```python
from build123d import *

# Parameters (mm, degrees)
CHAMFER1_SIZE = 0.2


with BuildPart() as part:
    # Sketch1 → Revolve1 (revolve)
    with BuildSketch(Plane.XY, mode=Mode.PRIVATE) as revolve1_sk:
        with BuildLine():
            Line((2.38125, 3.495554014), (2.38125, 2.495554014))
            Line((2.38125, 2.495554014), (4.7625, 2.495554014))
            Line((4.7625, 2.495554014), (4.7625, 0))
            Line((4.7625, 0), (2.38125, 0))
            Line((2.38125, 0), (2.38125, -11.43))
            Line((2.38125, -11.43), (0, -11.43))
            Line((0, -11.43), (0, 12.3825))
            ThreePointArc((0, 12.3825), (4.600221748, 8.852625702), (2.38125, 3.495554014))
        make_face()
    revolve(revolve1_sk.sketch.rotate(Axis((0, 48.717648678, 0), (0, -1, 0)), 180), axis=Axis((0, 48.717648678, 0), (0, -1, 0)))  # turned: the seam where the file's is

    # Chamfer1
    chamfer1_edges = [part.edges().sort_by_distance(p)[0] for p in [
        (2.38125, -11.43, 0),
        (4.7625, 0, 0),
        (4.7625, 2.495554014, 0),
    ]]
    chamfer(chamfer1_edges, length=CHAMFER1_SIZE)


solid = part.part
```
Design review of the part built by this model. Coordinates are the model's own, in mm. A direction names the side the tool comes from. Round coordinates to 2 decimals unless told otherwise and drop trailing zeros. Write each loop counter-clockwise with the first axis right and the second up, starting at its lowest first coordinate (ties: lowest second). Pieces come first, ordered by that corner, then holes. Notation, with made-up numbers: (28, 56.25) -> (55, 56.25) arc R16 ccw to (55, 76.25) -> close; hole circle Ø10 at (29, 10.25). An arc over 180 degrees is marked (long way). Write item = value, one per line. Start each with the question number.
1) Take a section at D-D, the plane y = 2. State the section outline as (x, z) points (1 decimal).
2) Clearance check with flat-ended pins moving along their axes: pin 1 (1 mm diameter, centred on x = -1.5, z = -3, fed in from -Y); pin 2 (3 mm diameter, centred on y = -7, z = -1, fed in from +X); pin 3 (2 mm diameter, centred on y = 5.5, z = 3, fed in from -X). State where each tip first meets the part, or that it passes through.
3) Wall thickness on probe 1 along Y at (x, z) = (-3, 2); probe 2 along Y at (x, z) = (2.75, -2.5); probe 3 along Z at (x, y) = (-2.5, 9.5): over which ranges is each line inside the solid? List them lowest first. Write a range as from..to.
4) Tool access review of faces 1 (the face through (2, 2.496, 2)), 2 (the face through (1.03, 1.23, 4.65)), 3 (the face through (-2, 0, 2)): name each direction out of +Z, -Z, +X, -X, +Y, -Y from which nothing blocks a thin tool from reaching the whole face with its end or side.
5) Take a section at C-C, the plane y = -2. State the section outline as (x, z) points, plus the area to 3 significant figures.
6) Mouldability with a two-part tool opening along Y and no side actions: class faces 4 (the face through (0, -11.43, 0)), 5 (the face through (0.516, 2.989, 2.325)), 6 (the face through (0.516, -5.694, 2.325)) as +Y half, -Y half, draft (parallel to the pull), parting line (faces both ways), or undercut.
Results list:
q1.outline = circle Ø9.5 at (0, 0)
q2.pin_1 = 0
q2.pin_2 = 2.38
q2.pin_3 = -3.94
q3.probe_1 = 0..2.5, 4.51..10.73
q3.probe_2 = 0..2.5, 4.64..10.6
q3.probe_3 = -3.59..3.59
q4.face_1 = none
q4.face_2 = +Y, -Y
q4.face_3 = -Y
q5.outline = circle Ø4.76 at (0, 0)
q5.area = 17.8 mm²
q6.face_4 = -Y half
q6.face_5 = undercut
q6.face_6 = draft
